Verification items for the finished model (mm, model axes). Face numbers are marked on the shaded views. A direction names the side the tool comes from. Coordinates: 2 decimals unless noted, no trailing zeros. Order: outer loops, then holes, each group sorted by start corner. A loop starts at its lowest first (then second) coordinate and runs counter-clockwise, first axis right, second up. Notation, with made-up numbers: M 57.25,65 L 97.25,65 A32 cw 97.25,99 Z; hole C 16,6.25 d5. An arc over 180 degrees is marked long. Return JSON: item names as keys, results as strings. Group by question number.
Q1. Mould release check, pull along X, two halves, no side actions. Record for the marked faces 3 and 4: pulls with the +X half, pulls with the -X half, needs draft (parallel to the pull), parting line crosses it, or undercut.
Q2. Section check B-B, the plane z = 13.5. Enter the section's corners in (x, y), then the cut area to 3 significant figures.
Q3. Go/stop test with flat-tipped pins: pin 1 Ø3 at (x, y) = (-39.5, -28) entering from +Z; pin 2 Ø5 at (x, y) = (-31.5, 5.5) entering from +Z; pin 3 Ø11.5 at (x, z) = (-15.5, 25) entering from +Y; pin 4 Ø8 at (x, z) = (-23.5, 27.5) entering from +Y. Record where each tip stops, or that it passes through.
Q4. Section check A-A, the plane z = 22.5. Enter the section's corners in (x, y), then the cut area to 3 significant figures.
Q5. Access from +Z, -Z, +X, -X, +Y, -Y to the whole of each face (thin tool, end or side, straight path). Record for the marked faces 1 and 2.
Q6. Section check C-C, the plane y = 5. Enter the section's corners in (x, z), then the cut area to 3 significant figures.
Q7. Section check D-D, the plane x = 17. Enter the section's corners in (y, z), then the cut area to 3 significant figures.
Q8. Thickness scan on probe 1 along Z at (x, y) = (10, 25); probe 2 along Y at (x, z) = (-15.5, 26.5); probe 3 along X at (y, z) = (-3.5, 12). Record the ranges inside material, lowest first.
Solid Edge part; units mm, degrees
sketch "Sketch1" plane through (0, 0, 0) normal (0, 0, 1) x (1, 0, 0)
  line L0 (-50.4769, -0.1262) -> (-31.3427, -46.3202)
  line L1 (-31.3427, -46.3202) -> (-10.2002, -25.1777)
  line L2 (-10.2002, -25.1777) -> (-24.3402, -25.1777)
  line L3 (-24.3402, -25.1777) -> (26.5942, 25.7567)
  line L4 (26.5942, 25.7567) -> (19.5231, 32.8278)
  line L5 (19.5231, 32.8278) -> (-26.4388, -13.1341)
  line L6 (-26.4388, -13.1341) -> (-50.4769, -0.1262)
  dimension "D1" = 50.4769
  dimension "D2" = 31.3427
  dimension "D3" = 26.5942
  dimension "D4" = 19.5231
  dimension "D5" = 10.2002
extrude "Protrusion1" add sketch "Sketch1" along normal blind 35
sketch "Sketch2" plane through (-12.0121, -6.8169, 0) normal (0, 0, -1) x (-0.8795, 0.4759, 0)
  line L0 (-1.7996, -43.9425) -> (-10.3318, -15.2857)
  line L1 (-10.3318, -15.2857) -> (2.1041, -22.0153)
  line L2 (2.1041, -22.0153) -> (-18.451, 47.0217)
  line L3 (-18.451, 47.0217) -> (6.4693, 54.4415)
  line L4 (6.4693, 54.4415) -> (28.4484, -19.3779)
  line L5 (28.4484, -19.3779) -> (-1.7996, -43.9425)
extrude "Extrusionsausprägung_6" add sketch "Sketch2" against normal blind 4
sketch "Sketch3" plane through (-3.4579, 9.8468, 19.5) normal (-0.7071, 0.7071, 0) x (0, 0, 1)
  circle A0 centre (-6.5, 10.45) radius 3.5
  circle A1 centre (-6.5, -19.55) radius 3.5
  dimension "D1" = 6.5
extrude "Cutout1" cut sketch "Sketch3" against normal through all
properties material "Nylon, allgemein"
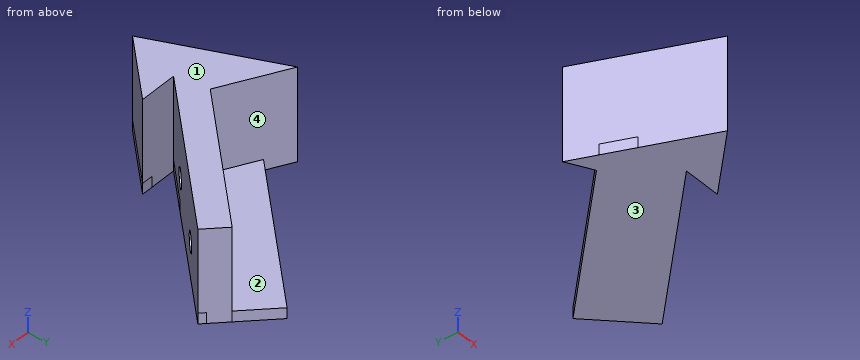
Numbers:
{
 "1": {"face 3": "needs draft", "face 4": "undercut"},
 "2": {"outline": "M -50.48,-0.13 L -31.34,-46.32 L -10.2,-25.18 L -24.34,-25.18 L -12.66,-13.5 L -19.73,-6.43 L -26.44,-13.13 Z; M -14.83,-1.53 L -7.76,-8.6 L 8.55,7.72 L 1.48,14.79 Z; M 6.38,19.69 L 13.45,12.61 L 26.59,25.76 L 19.52,32.83 Z", "area": "1,190 mm2"},
 "3": {"pin 1": "stops at z = 35", "pin 2": "stops at z = 4", "pin 3": "stops at y = 3.55", "pin 4": "stops at y = -6.2"},
 "4": {"outline": "M -50.48,-0.13 L -31.34,-46.32 L -10.2,-25.18 L -24.34,-25.18 L 26.59,25.76 L 19.52,32.83 L -26.44,-13.13 Z", "area": "1,330 mm2"},
 "5": {"face 1": "+Z, +X, -X, +Y, -Y", "face 2": "+Z, +Y"},
 "6": {"outline": "M -30.93,0 L 5.84,0 L 5.84,35 L -8.3,35 L -8.3,4 L -30.93,4 Z", "area": "585 mm2"},
 "7": {"outline": "M 16.16,0 L 35.35,0 L 35.35,4 L 30.3,4 L 30.3,35 L 16.16,35 Z", "area": "515 mm2"},
 "8": {"probe 1": "z = 0 to 4", "probe 2": "y = -30.48 to -25.18, -16.34 to -2.2", "probe 3": "x = -49.08 to -44.24, -13.02 to -2.66"}
}
